The listing builds one solid part. Answer for the finished solid, in the listing's coordinates (mm). Face numbers are marked on the shaded views. A direction names the side the tool comes from. Round coordinates to 2 decimals unless told otherwise and drop trailing zeros. Loops run counter-clockwise (first coordinate to the right, second up) from the corner with the lowest first, then second, coordinate; pieces in that order, holes last. Notation, with made-up numbers: (8.25, -38) - (40.25, -38) arc R23 cw to (40.25, -25) - close; hole circle Ø1 at (12, 29.25). An arc over 180 degrees is marked (long way). One line per item, written item: value.
```python
from build123d import *

# Parameters (mm, degrees)
BOSS_EXTRUDE1_DEPTH      = 101.6
SKETCH4_R                = 38.1
CUT_EXTRUDE1_DEPTH       = 20.32
BOSS_EXTRUDE3_DEPTH      = 10.16
BOSS_EXTRUDE3_DEPTH_BACK = 71.12
SKETCH5_R                = 4.993753619
BOSS_EXTRUDE4_DEPTH      = 5.08
BOSS_EXTRUDE4_DEPTH_BACK = 86.36
SKETCH6_R                = 2.54
SKETCH8_R                = 19.05
CUT_EXTRUDE2_DEPTH       = 3.175
SKETCH9_W                = 204.446341232
SKETCH9_H                = 212.005576541
CUT_EXTRUDE3_DEPTH       = 38.1
SKETCH10_W               = 191.95217793
SKETCH10_H               = 158.555264397
CUT_EXTRUDE4_DEPTH       = 6.096
SKETCH11_W               = 128.165166247
SKETCH11_H               = 88.990153167
CUT_EXTRUDE5_DEPTH       = 56.134
SKETCH12_W               = 45.159356145
SKETCH12_H               = 41.954498612
SKETCH12_W_2             = 24.473457524
SKETCH12_H_2             = 41.272764935
SKETCH12_H_3             = 38.685517003
BOSS_EXTRUDE5_DEPTH      = 10.414


with BuildPart() as part:
    # Sketch1 → Boss-Extrude1 (new body)
    with BuildSketch(Plane(origin=(0, 0, 0), x_dir=(1, 0, 0), z_dir=(0, 1, 0))):
        with BuildLine():
            Line((-91.44, 50.8), (91.44, 50.8))
            ThreePointArc((91.44, 50.8), (98.624204897, 47.824204897), (101.6, 40.64))
            Line((101.6, 40.64), (101.6, -40.64))
            ThreePointArc((101.6, -40.64), (98.624204897, -47.824204897), (91.44, -50.8))
            Line((91.44, -50.8), (-91.44, -50.8))
            ThreePointArc((-91.44, -50.8), (-98.624204897, -47.824204897), (-101.6, -40.64))
            Line((-101.6, -40.64), (-101.6, 40.64))
            ThreePointArc((-101.6, 40.64), (-98.624204897, 47.824204897), (-91.44, 50.8))
        make_face()
    extrude(amount=BOSS_EXTRUDE1_DEPTH)

    # Sketch4 → Cut-Extrude1 (cut)
    with BuildSketch(Plane(origin=(0, 0, -50.8), x_dir=(-1, 0, 0), z_dir=(0, 0, -1))):
        with Locations((-45.716232369, 0)):
            Circle(SKETCH4_R)
    cut_extrude1 = extrude(amount=-CUT_EXTRUDE1_DEPTH, mode=Mode.SUBTRACT)

    # Mirror1: Cut-Extrude1 across plane
    add(cut_extrude1.mirror(Plane.XY), mode=Mode.SUBTRACT)

    # Sketch5 → Boss-Extrude3 (add, two sides: drawn at the far end of the back side and taken through both)
    with BuildSketch(Plane(origin=(0, 0, -30.48), x_dir=(-1, 0, 0), z_dir=(0, 0, -1)).offset(-BOSS_EXTRUDE3_DEPTH_BACK)):
        with Locations((-45.716232369, 0)):
            Circle(SKETCH5_R)
    extrude(amount=BOSS_EXTRUDE3_DEPTH + BOSS_EXTRUDE3_DEPTH_BACK)

    # Sketch6 → Boss-Extrude4 (add, two sides: drawn at the far end of the back side and taken through both)
    with BuildSketch(Plane(origin=(0, 0, -40.64), x_dir=(-1, 0, 0), z_dir=(0, 0, -1)).offset(-BOSS_EXTRUDE4_DEPTH_BACK)):
        with Locations((-45.716232369, 0)):
            Circle(SKETCH6_R)
    extrude(amount=BOSS_EXTRUDE4_DEPTH + BOSS_EXTRUDE4_DEPTH_BACK)

    # Sketch8 → Cut-Extrude2 (cut)
    with BuildSketch(Plane(origin=(0, 0, 0), x_dir=(1, 0, 0), z_dir=(0, 1, 0))):
        with Locations(Location((-63.77539901, 0, 0), (0, 0, 270))):
            Circle(SKETCH8_R)
    extrude(amount=CUT_EXTRUDE2_DEPTH, mode=Mode.SUBTRACT)

    # Sketch9 → Cut-Extrude3 (cut)
    with BuildSketch(Plane(origin=(-101.6, 101.6, 0), x_dir=(0, 0, 1), z_dir=(-0.7071067811865512, 0.7071067811865438, 0))):
        with Locations((0, 45.254668325)):
            Rectangle(SKETCH9_W, SKETCH9_H)
    extrude(amount=-CUT_EXTRUDE3_DEPTH, mode=Mode.SUBTRACT)

    # Sketch10 → Cut-Extrude4 (cut)
    with BuildSketch(Plane(origin=(101.6, 101.6, 0), x_dir=(0, 0, -1), z_dir=(-0.7071067811865512, -0.7071067811865438, 0))):
        with Locations((0, 44.355551834)):
            Rectangle(SKETCH10_W, SKETCH10_H)
    extrude(amount=CUT_EXTRUDE4_DEPTH, mode=Mode.SUBTRACT)

    # Sketch11 → Cut-Extrude5 (cut)
    with BuildSketch(Plane(origin=(0, 101.6, 0), x_dir=(1, 0, 0), z_dir=(0, 1, 0))):
        with Locations((21.822922161, 0.221645033)):
            Rectangle(SKETCH11_W, SKETCH11_H)
    extrude(amount=-CUT_EXTRUDE5_DEPTH, mode=Mode.SUBTRACT)

    # Sketch12 → Boss-Extrude5 (add)
    with BuildSketch(Plane(origin=(0, 45.466, 0), x_dir=(1, 0, 0), z_dir=(0, 1, 0))):
        with Locations((-4.914184507, -1.800355644)):
            Rectangle(SKETCH12_W, SKETCH12_H)
        with Locations((63.116200395, 24.08033915)):
            Rectangle(SKETCH12_W_2, SKETCH12_H_2)
        with Locations((63.116200395, -24.930673049)):
            Rectangle(SKETCH12_W_2, SKETCH12_H_3)
    extrude(amount=BOSS_EXTRUDE5_DEPTH)


solid = part.part
```
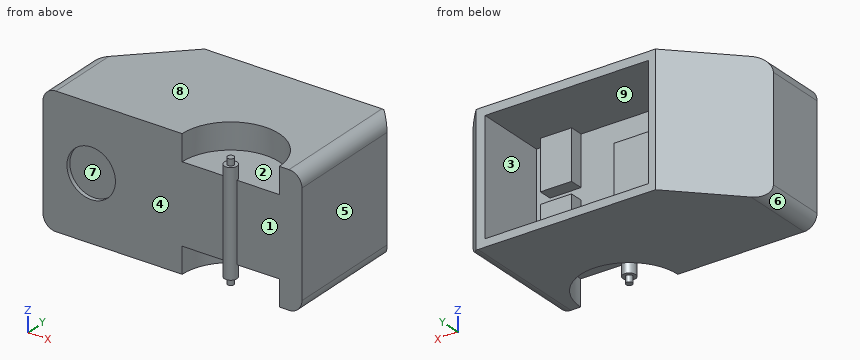
1) For the marked faces 1, 2, 3, 4 and 5, determine the directions among +Z, -Z, +X, -X, +Y, -Y from which every point of the face is accessible in a straight line to the end or side of a thin tool.
Final values:
face 1: +Z, -Z, +X, -Y
face 2: +Z
face 3: +Y
face 4: +Z, -Z, -X, -Y
face 5: +Z, -Z, +X, +Y, -Y
2) A cutting plane is placed at C-C on x = -35. Give the vertices of the cut face in (y, z), and give its area (3 significant figures).
Final values:
outline: (0, -50.8) - (101.6, -50.8) - (101.6, -44.72) - (45.47, -44.72) - (45.47, 44.27) - (101.6, 44.27) - (101.6, 50.8) - (0, 50.8) - close
area: 5,330 mm2
3) Consider L1, parallel to Z at x = 82.5, y = 80; L2, parallel to X at y = 1.9, z = 0; L3, parallel to X at y = 52, z = 18. Determine where each line is inside the solid, lowest interval first.
Final values:
L1: -50.8 to -44.72, 44.27 to 50.8
L2: -101.6 to -82.83, -44.73 to 101.6
L3: -97.32 to -42.26, -27.49 to 17.67, 50.88 to 75.35, 85.91 to 101.6
4) A cutting plane is placed at D-D on z = 0. Give the vertices of the cut face in (x, y) (1 decimal).
Final values:
outline: (-101.6, 0) - (-82.8, 0) - (-82.8, 3.2) - (-44.7, 3.2) - (-44.7, 0) - (40.7, 0) arc R5 ccw to (50.7, 0) - (101.6, 0) - (101.6, 93) - (93, 101.6) - (85.9, 101.6) - (85.9, 45.5) - (17.7, 45.5) - (17.7, 55.9) - (-27.5, 55.9) - (-27.5, 45.5) - (-42.3, 45.5) - (-42.3, 101.6) - (-47.7, 101.6) - (-101.6, 47.7) - close
5) Each of these flat-tipped pins is pushed along its axis until it touches: pin 1 Ø2.5 at (x, y) = (46.5, -1) entering from +Z; pin 2 Ø2 at (x, y) = (47, 17.5) entering from -Z; pin 3 Ø11 at (x, y) = (47.5, -1) entering from -Z. Where does it stop, or does it pass through?
Final values:
pin 1: z = 45.72
pin 2: z = -30.48
pin 3: z = -45.72
6) For a pull along Z with two mould halves and no side action, classify the marked faces 6, 7, 8 and 9 as released by +Z, released by -Z, zero draft, split by the parting line, or undercut.
Final values:
face 6: released by -Z
face 7: undercut
face 8: released by +Z
face 9: undercut
7) A cutting plane is placed at B-B on y = 83. Give the vertices of the cut face in (x, z).
Final values:
outline: (-66.32, -50.8) - (91.44, -50.8) arc R10.16 ccw to (101.6, -40.64) - (101.6, 40.64) arc R10.16 ccw to (91.44, 50.8) - (-66.32, 50.8) - close; hole (-42.26, -44.72) - (85.91, -44.72) - (85.91, 44.27) - (-42.26, 44.27) - close
8) A cutting plane is placed at A-A on z = -34.5. Give the vertices of the cut face in (x, y).
Final values:
outline: (-101.6, 0) - (7.62, 0) arc R38.1 cw to (83.82, 0) - (101.6, 0) - (101.6, 92.98) - (92.98, 101.6) - (85.91, 101.6) - (85.91, 45.47) - (75.35, 45.47) - (75.35, 55.88) - (50.88, 55.88) - (50.88, 45.47) - (-42.26, 45.47) - (-42.26, 101.6) - (-47.72, 101.6) - (-101.6, 47.72) - close; circle Ø9.99 at (45.72, 0)
